```python
from build123d import *

# Parameters (mm, degrees)
BOSS_EXTRUDE1_OUTLINE_R                    = 9.950311947
BOSS_EXTRUDE1_DEPTH                        = 3
SKETCH2_R                                  = 1.5
CUT_EXTRUDE1_DEPTH                         = 104
MIRROR1_AT_THE_SECOND_PLANE_COPY_1_SKETC_R = 1.5
MIRROR1_AT_THE_SECOND_PLANE_COPY_1_DEPTH   = 104
SKETCH3_R                                  = 1.5
CUT_EXTRUDE2_DEPTH                         = 104
MIRROR2_AT_THE_SECOND_PLANE_COPY_1_SKETC_R = 1.5
MIRROR2_AT_THE_SECOND_PLANE_COPY_1_DEPTH   = 104
FILLET1_R                                  = 20


# Read off the part's stored shape, not the designer's step: Boss-Extrude1
with BuildPart() as part:
    # Boss-Extrude1 outline → Boss-Extrude1 (new body)
    with BuildSketch(Plane.XY):
        Polygon((28.786796564, 44.142135624), (28.786796564, 90), (-28.786796564, 90), (-28.786796564, 44.142135624), (-50, 22.928932188), (-50, -22.928932188), (-28.786796564, -44.142135624), (-28.786796564, -90), (28.786796564, -90), (28.786796564, -44.142135624), (50, -22.928932188), (50, 22.928932188), align=None)
        Circle(BOSS_EXTRUDE1_OUTLINE_R, mode=Mode.SUBTRACT)
    extrude(amount=BOSS_EXTRUDE1_DEPTH)

    # Sketch2 → Cut-Extrude1 (cut, through all)
    with BuildSketch(Plane.XY.offset(3)):
        with Locations((-28.786796564, 32.928932188)):
            Circle(SKETCH2_R)
        with Locations((-18.786796564, 22.928932188)):
            Circle(SKETCH2_R)
        with Locations((-28.786796564, 12.928932188)):
            Circle(SKETCH2_R)
        with Locations((-38.786796564, 22.928932188)):
            Circle(SKETCH2_R)
    cut_extrude1 = extrude(amount=-CUT_EXTRUDE1_DEPTH, mode=Mode.SUBTRACT)

    # Mirror1: Cut-Extrude1 across plane
    add(cut_extrude1.mirror(Plane(origin=(0, 0, 0), x_dir=(0, 0, 1), z_dir=(1, 0, 0))), mode=Mode.SUBTRACT)

    # Mirror1 at the second plane: Cut-Extrude1 across plane
    add(cut_extrude1.mirror(Plane.ZX), mode=Mode.SUBTRACT)

    # Mirror1 at the second plane copy 1 sketc → Mirror1 at the second plane copy 1 (cut, through all)
    with BuildSketch(Plane(origin=(0, 0, 3), x_dir=(-1, 0, 0), z_dir=(0, 0, 1))):
        with Locations((-28.786796564, 32.928932188)):
            Circle(MIRROR1_AT_THE_SECOND_PLANE_COPY_1_SKETC_R)
        with Locations((-18.786796564, 22.928932188)):
            Circle(MIRROR1_AT_THE_SECOND_PLANE_COPY_1_SKETC_R)
        with Locations((-28.786796564, 12.928932188)):
            Circle(MIRROR1_AT_THE_SECOND_PLANE_COPY_1_SKETC_R)
        with Locations((-38.786796564, 22.928932188)):
            Circle(MIRROR1_AT_THE_SECOND_PLANE_COPY_1_SKETC_R)
    extrude(amount=-MIRROR1_AT_THE_SECOND_PLANE_COPY_1_DEPTH, mode=Mode.SUBTRACT)

    # Sketch3 → Cut-Extrude2 (cut, through all)
    with BuildSketch(Plane.XY.offset(3)):
        with Locations((0, 85)):
            Circle(SKETCH3_R)
        with Locations((-23.786796564, 66.575)):
            Circle(SKETCH3_R)
        with Locations((-45, 0)):
            Circle(SKETCH3_R)
    cut_extrude2 = extrude(amount=-CUT_EXTRUDE2_DEPTH, mode=Mode.SUBTRACT)

    # Mirror2: Cut-Extrude2 across plane
    add(cut_extrude2.mirror(Plane(origin=(0, 0, 0), x_dir=(0, 0, 1), z_dir=(1, 0, 0))), mode=Mode.SUBTRACT)

    # Mirror2 at the second plane: Cut-Extrude2 across plane
    add(cut_extrude2.mirror(Plane.ZX), mode=Mode.SUBTRACT)

    # Mirror2 at the second plane copy 1 sketc → Mirror2 at the second plane copy 1 (cut, through all)
    with BuildSketch(Plane(origin=(0, 0, 3), x_dir=(-1, 0, 0), z_dir=(0, 0, 1))):
        with Locations((0, 85)):
            Circle(MIRROR2_AT_THE_SECOND_PLANE_COPY_1_SKETC_R)
        with Locations((-23.786796564, 66.575)):
            Circle(MIRROR2_AT_THE_SECOND_PLANE_COPY_1_SKETC_R)
        with Locations((-45, 0)):
            Circle(MIRROR2_AT_THE_SECOND_PLANE_COPY_1_SKETC_R)
    extrude(amount=-MIRROR2_AT_THE_SECOND_PLANE_COPY_1_DEPTH, mode=Mode.SUBTRACT)

    # Fillet1
    fillet1_edges = [part.edges().sort_by_distance(p)[0] for p in [
        (28.786796564, 44.142135624, 1.5),
        (50, 22.928932188, 1.5),
        (50, -22.928932188, 1.5),
        (28.786796564, -44.142135624, 1.5),
        (28.786796564, -90, 1.5),
        (-28.786796564, -90, 1.5),
        (-28.786796564, -44.142135624, 1.5),
        (-50, -22.928932188, 1.5),
        (-50, 22.928932188, 1.5),
        (-28.786796564, 44.142135624, 1.5),
        (-28.786796564, 90, 1.5),
        (28.786796564, 90, 1.5),
    ]]
    fillet(fillet1_edges, radius=FILLET1_R)


solid = part.part
```
The model under review builds one solid part; all positions refer to its coordinate system, in mm. Round coordinates to 2 decimals unless told otherwise and drop trailing zeros. Order: outer loops, then holes, each group sorted by start corner. A loop starts at its lowest first (then second) coordinate and runs counter-clockwise, first axis right, second up. Notation, with made-up numbers: (86, 20.25) -> (94, 20.25) arc R8 cw to (94, 30.25) -> close; hole circle Ø4 at (30, 7.25). An arc over 180 degrees is marked (long way). One line per item, written item: value. Start each with the question number.
Q1. Take a section at C-C (x = -5). Write out the cut boundary in (y, z), and give its area (3 significant figures).
Q2. Take a section at B-B (y = 49). Write out the cut boundary in (x, z), and give its area (3 significant figures).
Q3. Wall thickness on line 1 (Y direction, x = 0, z = 0.95); line 2 (Y direction, x = 20, z = 0.45); line 3 (X direction, y = 22, z = 2.2): over which ranges is each line inside the solid? List them lowest first.
Q4. Take a section at A-A (x = 7). Write out the cut boundary in (y, z), and give its area (3 significant figures).
Q5. Take a section at D-D (z = 1.1). Count the separate pieces of the cut face and the enclosed holes in it, and give its area (3 significant figures).
Q6. Clearance check with flat-ended pins moving along their axes: pin 1 Ø1.8 at (x, y) = (-18.79, -22.93) entering from -Z; pin 2 Ø4 at (x, y) = (28.79, 32.93) entering from +Z; pin 3 Ø1.5 at (y, z) = (-57.5, 1.5) entering from -X. State where each tip first meets the part, or that it passes through.
Q7. Mouldability with a two-part tool opening along X and no side actions: class faces 1 (the face through (-1.295, 9.866, 1.479)), 2 (the face through (-22.77, -84.3, 1.52)), 3 (the face through (10.4, 1.3, 0)) as released by +X, released by -X, zero draft, split by the parting line, or undercut.
Reported:
1. outline: (-90, 0) -> (-8.6, 0) -> (-8.6, 3) -> (-90, 3) -> close; (8.6, 0) -> (90, 0) -> (90, 3) -> (8.6, 3) -> close
1. area: 488 mm2
2. outline: (-29.08, 0) -> (29.08, 0) -> (29.08, 3) -> (-29.08, 3) -> close
2. area: 174 mm2
3. line 1: y = -90 to -86.5, -83.5 to -9.95, 9.95 to 83.5, 86.5 to 90
3. line 2: y = -86.56 to -23.81, -22.05 to 22.05, 23.81 to 86.56
3. line 3: x = -48.6 to -39.96, -37.61 to -19.96, -17.61 to 17.61, 19.96 to 37.61, 39.96 to 48.6
4. outline: (-90, 0) -> (-7.07, 0) -> (-7.07, 3) -> (-90, 3) -> close; (7.07, 0) -> (90, 0) -> (90, 3) -> (7.07, 3) -> close
4. area: 498 mm2
5. separate pieces: 1
5. enclosed holes: 25
5. area: 12,400 mm2
6. pin 1: passes through
6. pin 2: stops at z = 3
6. pin 3: stops at x = -28.79
7. face 1: undercut
7. face 2: released by -X
7. face 3: zero draft
